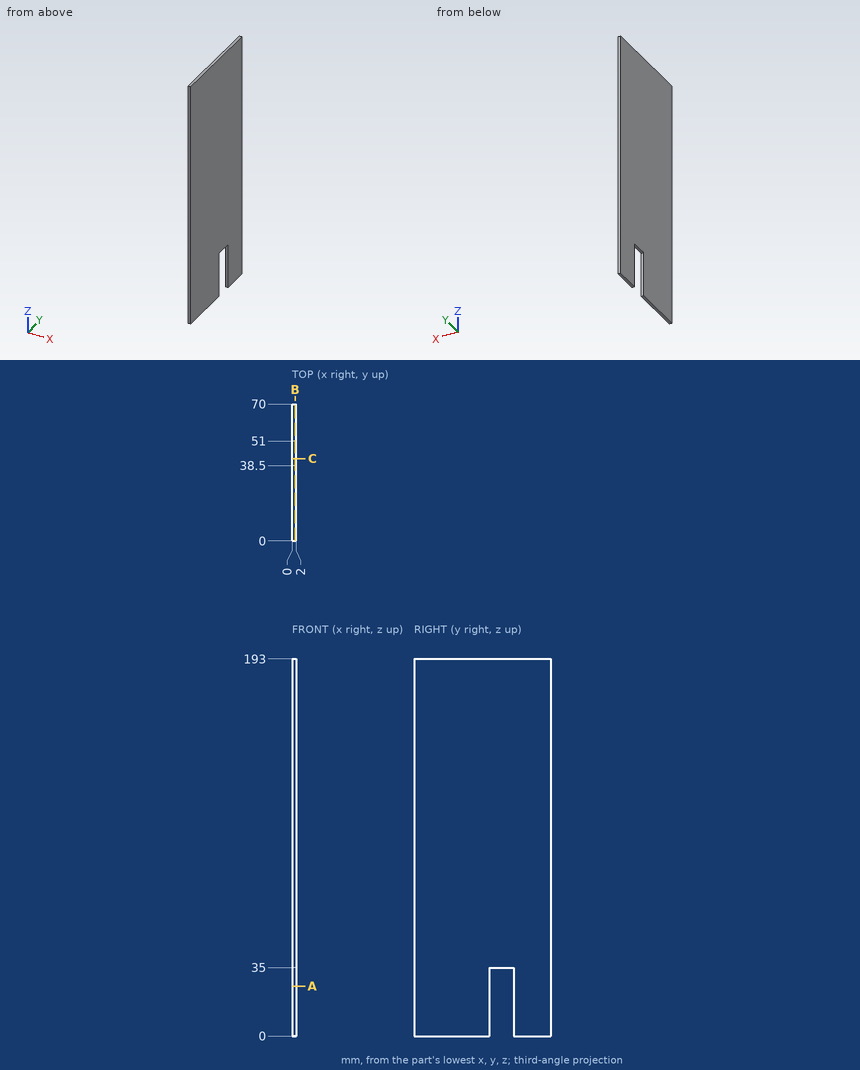
For this review, use the dimensioned drawing (mm, ordinates from the lowest corner) and the shaded views. Give positions to 0.01 mm unless a question says otherwise; leave off trailing zeros. Order: outer loops, then holes, each group sorted by start corner. A loop starts at its lowest first (then second) coordinate and runs counter-clockwise, first axis right, second up.
1) Take a section at C-C (y = 42). Give the boundary of the cut face in (x, z).
2) Wall thickness on line 1 (Y direction, x = 0.85, z = 11); line 2 (Z direction, x = 1.35, y = 43.5): over which ranges is each line inside the solid? List them lowest first.
3) Take a section at B-B (x = 1.5). Give the boundary of the cut face in (y, z), then the cut area to 3 significant figures.
4) Take a section at A-A (z = 25.5). Give the boundary of the cut face in (x, y).
5) Insertion check: pin 1 (1 mm diameter, centred on x = 1, y = 46.5, fed in from -Z). The pin has a flat end and moves straight along its axis. Give the tip position at first contact, or say it passes through.
Derived:
1. outline: (0, 35) - (2, 35) - (2, 193) - (0, 193) - close
2. line 1: y = 0 to 38.5, 51 to 70
2. line 2: z = 35 to 193
3. outline: (0, 0) - (38.5, 0) - (38.5, 35) - (51, 35) - (51, 0) - (70, 0) - (70, 193) - (0, 193) - close
3. area: 13,100 mm2
4. outline: (0, 0) - (2, 0) - (2, 38.5) - (0, 38.5) - close; (0, 51) - (2, 51) - (2, 70) - (0, 70) - close
5. pin 1: stops at z = 35
